from build123d import *

# Parameters (mm, degrees)
SKETCH1_W                  = 12.065
SKETCH1_H                  = 4.445
BASE_DEPTH                 = 15.875
SKETCH7_W                  = 6.35
SKETCH7_H                  = 10.16
BOSS_EXTRUDE1_DEPTH        = 11.43
SKETCH3_R                  = 1.27
SHAFTHOLE_DEPTH            = 22.78984712
F_4_40_TAPPED_HOLE1_REACH  = 25.247
F_4_40_TAPPED_HOLE1_BORE_R = 1.1303
CHAMFER1_SIZE              = 5.715


with BuildPart() as part:
    # Sketch1 → Base (new body)
    with BuildSketch(Plane.XY):
        Rectangle(SKETCH1_W, SKETCH1_H)
    extrude(amount=BASE_DEPTH)

    # Sketch7 → Boss-Extrude1 (add)
    with BuildSketch(Plane(origin=(0, 2.2225, 0), x_dir=(1, 0, 0), z_dir=(0, 1, 0))):
        with Locations((0, -5.08)):
            Rectangle(SKETCH7_W, SKETCH7_H)
    extrude(amount=BOSS_EXTRUDE1_DEPTH)

    # Sketch3 → ShaftHole (cut, through all)
    with BuildSketch(Plane(origin=(0, 0, 0), x_dir=(-1, 0, 0), z_dir=(0, 0, -1))):
        with Locations((0, 9.525)):
            Circle(SKETCH3_R)
    extrude(amount=-SHAFTHOLE_DEPTH, mode=Mode.SUBTRACT)

    # #4-40 Tapped Hole1 bore → #4-40 Tapped Hole1 (cut, up to next)
    with BuildSketch(Plane(origin=(0, 13.6525, 0), x_dir=(1, 0, 0), z_dir=(0, 1, 0)), mode=Mode.PRIVATE) as f_4_40_tapped_hole1_sk1:
        with Locations((0, -2.54)):
            Circle(F_4_40_TAPPED_HOLE1_BORE_R)
    f_4_40_tapped_hole1_tool1 = extrude(f_4_40_tapped_hole1_sk1.sketch, amount=-F_4_40_TAPPED_HOLE1_REACH, mode=Mode.PRIVATE) & part.part
    add(f_4_40_tapped_hole1_tool1.solids().sort_by_distance((0, 13.6525, 2.54))[0], mode=Mode.SUBTRACT)

    # Chamfer1
    chamfer1_edges = [part.edges().sort_by_distance(p)[0] for p in [
        (0, 2.2225, 10.16),
    ]]
    chamfer(chamfer1_edges, length=CHAMFER1_SIZE - 0.0001)  # a hair under: the kernel refuses the full size


solid = part.part
Build history of the part. All positions in model axes, mm. A direction names the side the tool comes from. Round coordinates to 2 decimals unless told otherwise and drop trailing zeros. Loops run counter-clockwise (first coordinate to the right, second up) from the corner with the lowest first, then second, coordinate; pieces in that order, holes last. Notation, with made-up numbers: (88, -39.75) -> (122, -39.75) arc R30 cw to (122, -17.75) -> close; hole circle Ø8 at (11, 45.5). An arc over 180 degrees is marked (long way). Use CSV: the item, a comma, the result in double quotes. Start each with the question number.
Q1. Flat gauge pins, fed straight in: pin 1 Ø4.5 at (x, y) = (0.5, 11.5) entering from +Z; pin 2 Ø5.5 at (y, z) = (6, 10.5) entering from +X (3 decimals). Where does each tip first touch, or does it go through?
Q2. Saw through at A-A on x = 0. Count the separate pieces of the cut face and the enclosed holes in it, and give its area (3 significant figures).
Q3. Saw through at B-B on z = 2.54. Give the cut face in (x, y) (1 decimal), and give its area (3 significant figures).
Q4. Mould opens along X. For faces 6 (the face through (0.275, 8.285, 5.009)), 7 (the face through (4, 2.222, 8)), 8 (the face through (6.032, 0, 8)) say: +X half, -X half, draft (parallel to the pull), parting line (faces both ways), or undercut.
Q5. Which spindle directions (+Z, -Z, +X, -X, +Y, -Y) get a long thin tool onto all of the face, cutting with end or side? Do faces 1 (the face through (0, 4, 0)), 2 (the face through (1.08, 11.9, 2.2)), 3 (the face through (-3.175, 8, 6)), 4 (the face through (3.175, 8, 6)), 5 (the face through (0, 11, 10.16)). Say none if no direction does.
Q6. Saw through at C-C on y = 11.5. Give the cut face in (x, z) (3 decimals).
Q7. Drill centre lines: L1, parallel to X at y = 11.35, z = 2.54 (3 decimals); L2, parallel to Z at x = 0, y = 11.4; L3, parallel to Y at x = 0, z = 7 (1 decimal). Where is each one in solid material? Low to high.
Solutions:
1,pin 1,"stops at z = 10.16"
1,pin 2,"stops at x = 3.175"
2,separate pieces,"3"
2,enclosed holes,"0"
2,area,"171 mm^2"
3,outline,"(-6, -2.2) -> (6, -2.2) -> (6, 2.2) -> (3.2, 2.2) -> (3.2, 13.7) -> (1.1, 13.7) -> (1.1, 10.1) arc R1.3 cw (long way) to (-1.1, 10.1) -> (-1.1, 13.7) -> (-3.2, 13.7) -> (-3.2, 2.2) -> (-6, 2.2) -> close"
3,area,"114 mm^2"
4,face 6,"undercut"
4,face 7,"draft"
4,face 8,"+X half"
5,face 1,"-Z, +X, -X, +Y, -Y"
5,face 2,"+Y"
5,face 3,"+Z, -Z, -X, +Y"
5,face 4,"+Z, -Z, +X, +Y"
5,face 5,"+Z, +X, -X, +Y"
6,outline,"(-3.175, 0) -> (3.175, 0) -> (3.175, 10.16) -> (-3.175, 10.16) -> close; hole circle Ø2.261 at (0, 2.54)"
7,L1,"x = -3.175 to -1.13, 1.13 to 3.175"
7,L2,"z = 0 to 1.41, 3.67 to 10.16"
7,L3,"y = -2.2 to 8.3, 10.8 to 13.7"
